```python
from build123d import *

# Parameters (mm, degrees)
F1_DEPTH = 5
F2_DEPTH = 15


with BuildPart() as f1:
    # F0 (on Top) → F1 (new body)
    with BuildSketch(Plane.XY):
        with BuildLine():
            Line((1.5, -39.647717), (4.487062, -0.340988))
            ThreePointArc((4.487062, -0.340988), (0.169154, -4.49682), (-4.448765, -0.677121))
            Line((-4.448765, -0.677121), (-1.5, -39.647717))
            Line((-1.5, -39.647717), (1.5, -39.647717))
        make_face()
    extrude(amount=F1_DEPTH)

    # F0 (on Top) → F2 (join)
    with BuildSketch(Plane.XY):
        with BuildLine():
            ThreePointArc((4.487062, -0.340988), (4.496764, -0.170617), (4.5, 0))
            ThreePointArc((4.5, 0), (0, 4.5), (-4.5, 0))
            Line((-4.5, 0), (-4.448765, -0.677121))
            ThreePointArc((-4.448765, -0.677121), (0.169154, -4.49682), (4.487062, -0.340988))
        make_face()
    extrude(amount=F2_DEPTH)


solid = f1.part
```
Here's how the part is built. I have some questions about the finished solid (model axes, mm). A direction names the side the tool comes from. Give positions to 0.01 mm unless a question says otherwise; leave off trailing zeros. Order: outer loops, then holes, each group sorted by start corner. A loop starts at its lowest first (then second) coordinate and runs counter-clockwise, first axis right, second up. Notation, with made-up numbers: (36, 11) -> (58, 11) arc R14 ccw to (58, 19) -> close; hole circle Ø10 at (20, 31.25). An arc over 180 degrees is marked (long way). Use CSV: the item, a comma, the result in double quotes. Start each with the question number.
Item 1: Suppose I cut it at A-A (x = 0). List the corners of the cut face in (y, z) for me.
Item 2: Suppose I cut it at C-C (y = -29). List the corners of the cut face in (x, z) for me.
Item 3: If I drill on probe 1 along Z at (x, y) = (-0.75, -17.5); probe 2 along Y at (x, z) = (3.5, 14.25); probe 3 along Y at (x, z) = (1.5, 6), over which ranges is the centre line in solid material (lowest first)? Write a range as [from, to].
Item 4: On a 3-axis mill with a long thin cutter (end or side, diameter ignored), from which of +Z, -Z, +X, -X, +Y, -Y can I reach the whole of each face in a straight line? I mean faces 1 (the cylindrical face through (0.1, -4.5, 9.9)), 2 (the flat face through (0, -12, 0)). Say none if no direction works.
Item 5: Suppose I cut it at B-B (z = 2.5). List the corners of the cut face in (x, y) for me, and give its area (3 significant figures).
Item 6: Suppose I cut it at D-D (z = 5.5). List the corners of the cut face in (x, y) for me.
Item 7: I'm going to push flat-ended pins straight in: P1, Ø1, axis at x = 2, y = -16, coming from the +Z side; P2, Ø2, axis at x = -2, z = 13.5, coming from the -Y side; P3, Ø1.5, axis at x = 1.5, y = -2.5, coming from the -Z side; P4, Ø4, axis at y = -4, z = 8.5, coming from the +X side. Where does each tip first touch, or does it pass through?
Answer block:
1,outline,"(-39.65, 0) -> (4.5, 0) -> (4.5, 15) -> (-4.5, 15) -> (-4.5, 5) -> (-39.65, 5) -> close"
2,outline,"(-2.31, 0) -> (2.31, 0) -> (2.31, 5) -> (-2.31, 5) -> close"
3,probe 1,"z = [0, 5]"
3,probe 2,"y = [-2.83, 2.83]"
3,probe 3,"y = [-4.24, 4.24]"
4,face 1,"+Z, -Y"
4,face 2,"-Z, +X, -X, +Y, -Y"
5,outline,"(-4.5, 0) -> (-4.45, -0.68) -> (-1.5, -39.65) -> (1.5, -39.65) -> (4.49, -0.34) arc R4.5 ccw to (4.5, 0) arc R4.5 ccw to start"
5,area,"270 mm^2"
6,outline,"(-4.5, 0) -> (-4.45, -0.68) arc R4.5 ccw to (4.49, -0.34) arc R4.5 ccw to (4.5, 0) arc R4.5 ccw to start"
7,P1,"stops at z = 5"
7,P2,"stops at y = -4.39"
7,P3,"stops at z = 0"
7,P4,"stops at x = 4.03"
